from build123d import *

# Parameters (mm, degrees)
SKETCH1_W                = 16.6
SKETCH1_H                = 11.5
BOSS_EXTRUDE1_DEPTH      = 10
SKETCH2_W                = 21
SKETCH2_H                = 14.8
BOSS_EXTRUDE2_DEPTH      = 1.5
SKETCH3_W                = 0.5
SKETCH3_H                = 5
BOSS_EXTRUDE3_DEPTH      = 8
SKETCH4_W                = 0.5
SKETCH4_H                = 0.4
CUT_EXTRUDE1_DEPTH       = 17.75
BOSS_EXTRUDE4_START      = -5.75
SKETCH5_W                = 0.75
SKETCH5_H                = 2.5
BOSS_EXTRUDE4_DEPTH      = 11.5
BOSS_EXTRUDE5_DEPTH      = 2.8
BOSS_EXTRUDE5_DEPTH_BACK = 2.8
CHAMFER1_SIZE            = 1.8
CHAMFER1_SIZE2           = 1.039230485
BOSS_EXTRUDE6_DEPTH      = 4.65
SKETCH9_W                = 1.1
SKETCH9_H                = 0.45
BOSS_EXTRUDE7_DEPTH      = 1.9
CHAMFER2_SIZE            = 0.5
CHAMFER2_SIZE2           = 0.288675135
CHAMFER2_PART_2_SIZE     = 0.5
CHAMFER2_PART_2_SIZE2    = 0.288675135
CHAMFER2_PART_3_SIZE     = 0.5
CHAMFER2_PART_3_SIZE2    = 0.288675135
CHAMFER2_PART_4_SIZE     = 0.5
CHAMFER2_PART_4_SIZE2    = 0.288675135
CHAMFER2_PART_5_SIZE     = 0.5
CHAMFER2_PART_5_SIZE2    = 0.288675135
CHAMFER2_PART_6_SIZE     = 0.5
CHAMFER2_PART_6_SIZE2    = 0.288675135
CHAMFER2_PART_7_SIZE     = 0.5
CHAMFER2_PART_7_SIZE2    = 0.288675135
CHAMFER2_PART_8_SIZE     = 0.5
CHAMFER2_PART_8_SIZE2    = 0.288675135


with BuildPart() as part:
    # Sketch1 → Boss-Extrude1 (new body)
    with BuildSketch(Plane.XY):
        Rectangle(SKETCH1_W, SKETCH1_H)
    extrude(amount=BOSS_EXTRUDE1_DEPTH)

    # Sketch2 → Boss-Extrude2 (add)
    with BuildSketch(Plane.XY.offset(10)):
        Rectangle(SKETCH2_W, SKETCH2_H)
    extrude(amount=BOSS_EXTRUDE2_DEPTH)

    # Sketch3 → Boss-Extrude3 (add)
    with BuildSketch(Plane(origin=(0, 0, 0), x_dir=(-1, 0, 0), z_dir=(0, 0, -1))):
        with Locations((-6, 0)):
            Rectangle(SKETCH3_W, SKETCH3_H)
        Rectangle(SKETCH3_W, SKETCH3_H)
    extrude(amount=BOSS_EXTRUDE3_DEPTH)

    # Sketch4 → Cut-Extrude1 (cut, through all)
    with BuildSketch(Plane(origin=(6.25, 0, 0), x_dir=(0, 0, -1), z_dir=(1, 0, 0))):
        with Locations((2.25, 2.3)):
            Rectangle(SKETCH4_W, SKETCH4_H)
        with BuildLine():
            Line((0, 0.75), (0, -0.75))
            ThreePointArc((0, -0.75), (0.75, 0), (0, 0.75))
        make_face()
        Polygon((6.5, 2.5), (8, 1.449688693), (8, 2.5), align=None)
        with BuildLine():
            Line((5.432692308, 0.612598863), (6.3, 0))
            Line((6.3, 0), (5.432692308, -0.612598863))
            ThreePointArc((5.432692308, -0.612598863), (4.25, 0), (5.432692308, 0.612598863))
        make_face()
        Polygon((8, -2.5), (8, -1.449688693), (6.5, -2.5), align=None)
        with Locations((2.25, -2.3)):
            Rectangle(SKETCH4_W, SKETCH4_H)
    extrude(amount=-CUT_EXTRUDE1_DEPTH, mode=Mode.SUBTRACT)

    # Sketch5 → Boss-Extrude4 (add)
    with BuildSketch(Plane(origin=(0, 0, 0), x_dir=(1, 0, 0), z_dir=(0, 1, 0)).offset(BOSS_EXTRUDE4_START)):
        with Locations((-8.675, -1.25)):
            Rectangle(SKETCH5_W, SKETCH5_H)
    boss_extrude4 = extrude(amount=BOSS_EXTRUDE4_DEPTH)

    # Mirror1: Boss-Extrude4 across plane
    add(boss_extrude4.mirror(Plane(origin=(0, 0, 0), x_dir=(0, 0, 1), z_dir=(1, 0, 0))))

    # Sketch6 → Boss-Extrude5 (add, two sides)
    with BuildSketch(Plane(origin=(0, 0, 0), x_dir=(1, 0, 0), z_dir=(0, 1, 0))) as boss_extrude5_sk:
        with BuildLine():
            Line((-9.05, -2.5), (-10.124907983, -5.653347952))
            ThreePointArc((-10.124907983, -5.653347952), (-10.231819447, -6.312838644), (-10.115557515, -6.970745323))
            Line((-10.115557515, -6.970745323), (-9.056614332, -9.938626949))
            Line((-9.056614332, -9.938626949), (-9.034716365, -10))
            Line((-9.034716365, -10), (-8.3, -10))
            Line((-8.3, -10), (-8.3, -9.827371619))
            Line((-8.3, -9.827371619), (-8.350231447, -9.686588817))
            Line((-8.350231447, -9.686588817), (-9.438479941, -6.636573707))
            ThreePointArc((-9.438479941, -6.636573707), (-9.496610907, -6.307620368), (-9.443155175, -5.977875022))
            Line((-9.443155175, -5.977875022), (-8.34011069, -2.741985882))
            Line((-8.34011069, -2.741985882), (-8.3, -2.624317241))
            Line((-8.3, -2.624317241), (-8.3, -2.5))
            Line((-8.3, -2.5), (-9.05, -2.5))
        make_face()
        with BuildLine():
            Line((8.3, -9.827371619), (8.350231447, -9.686588817))
            Line((8.350231447, -9.686588817), (9.438479941, -6.636573707))
            ThreePointArc((9.438479941, -6.636573707), (9.496610907, -6.307620368), (9.443155175, -5.977875022))
            Line((9.443155175, -5.977875022), (8.34011069, -2.741985882))
            Line((8.34011069, -2.741985882), (8.3, -2.624317241))
            Line((8.3, -2.624317241), (8.3, -2.5))
            Line((8.3, -2.5), (9.05, -2.5))
            Line((9.05, -2.5), (10.124907983, -5.653347952))
            ThreePointArc((10.124907983, -5.653347952), (10.231819447, -6.312838644), (10.115557515, -6.970745323))
            Line((10.115557515, -6.970745323), (9.056614332, -9.938626949))
            Line((9.056614332, -9.938626949), (9.034716365, -10))
            Line((9.034716365, -10), (8.3, -10))
            Line((8.3, -10), (8.3, -9.827371619))
        make_face()
    extrude(amount=BOSS_EXTRUDE5_DEPTH)
    extrude(boss_extrude5_sk.sketch, amount=-BOSS_EXTRUDE5_DEPTH_BACK)

    # Chamfer1
    chamfer1_edges = [part.edges().sort_by_distance(p)[0] for p in [
        (10.5, 0, 11.5),
        (0, 7.4, 11.5),
        (-10.5, 0, 11.5),
        (0, -7.4, 11.5),
    ]]
    chamfer1_side = [part.faces().sort_by_distance(p)[0] for p in [
        (0, 0, 11.5),
    ]]
    chamfer(chamfer1_edges, length=CHAMFER1_SIZE, length2=CHAMFER1_SIZE2, reference=chamfer1_side[0])

    # Sketch7 → Boss-Extrude6 (add, symmetric)
    with BuildSketch(Plane(origin=(0, 0, 0), x_dir=(1, 0, 0), z_dir=(0, 1, 0))):
        with BuildLine():
            Line((-7.2, -11.5), (-3.398718251, -16.8))
            add(Edge.make_bspline(
                [(-3.398718251, -16.8), (0.927387699, -12.334784825), (7.2, -11.5)],
                knots=[0, 0, 0, 1, 1, 1], degree=2))
            Line((7.2, -11.5), (-7.2, -11.5))
        make_face()
    extrude(amount=BOSS_EXTRUDE6_DEPTH, both=True)

    # Sketch9 → Boss-Extrude7 (add)
    with BuildSketch(Plane(origin=(0, 0, 10), x_dir=(-1, 0, 0), z_dir=(0, 0, -1))):
        with Locations((-7.425, 5.975)):
            Rectangle(SKETCH9_W, SKETCH9_H)
        with Locations((-2.475, 5.975)):
            Rectangle(SKETCH9_W, SKETCH9_H)
        with Locations((2.475, 5.975)):
            Rectangle(SKETCH9_W, SKETCH9_H)
        with Locations((7.425, 5.975)):
            Rectangle(SKETCH9_W, SKETCH9_H)
        with Locations((7.425, -5.975)):
            Rectangle(SKETCH9_W, SKETCH9_H)
        with Locations((2.475, -5.975)):
            Rectangle(SKETCH9_W, SKETCH9_H)
        with Locations((-2.475, -5.975)):
            Rectangle(SKETCH9_W, SKETCH9_H)
        with Locations((-7.425, -5.975)):
            Rectangle(SKETCH9_W, SKETCH9_H)
    extrude(amount=BOSS_EXTRUDE7_DEPTH)

    # Chamfer2
    chamfer2_edges = [part.edges().sort_by_distance(p)[0] for p in [
        (7.425, 6.2, 8.1),
    ]]
    chamfer2_side = [part.faces().sort_by_distance(p)[0] for p in [
        (7.425, 6.2, 9.05),
    ]]
    chamfer(chamfer2_edges, length=CHAMFER2_SIZE, length2=CHAMFER2_SIZE2, reference=chamfer2_side[0])

    # Chamfer2 part 2
    chamfer2_part_2_edges = [part.edges().sort_by_distance(p)[0] for p in [
        (2.475, 6.2, 8.1),
    ]]
    chamfer2_part_2_side = [part.faces().sort_by_distance(p)[0] for p in [
        (2.475, 6.2, 9.05),
    ]]
    chamfer(chamfer2_part_2_edges, length=CHAMFER2_PART_2_SIZE, length2=CHAMFER2_PART_2_SIZE2, reference=chamfer2_part_2_side[0])

    # Chamfer2 part 3
    chamfer2_part_3_edges = [part.edges().sort_by_distance(p)[0] for p in [
        (-2.475, 6.2, 8.1),
    ]]
    chamfer2_part_3_side = [part.faces().sort_by_distance(p)[0] for p in [
        (-2.475, 6.2, 9.05),
    ]]
    chamfer(chamfer2_part_3_edges, length=CHAMFER2_PART_3_SIZE, length2=CHAMFER2_PART_3_SIZE2, reference=chamfer2_part_3_side[0])

    # Chamfer2 part 4
    chamfer2_part_4_edges = [part.edges().sort_by_distance(p)[0] for p in [
        (-7.425, 6.2, 8.1),
    ]]
    chamfer2_part_4_side = [part.faces().sort_by_distance(p)[0] for p in [
        (-7.425, 6.2, 9.05),
    ]]
    chamfer(chamfer2_part_4_edges, length=CHAMFER2_PART_4_SIZE, length2=CHAMFER2_PART_4_SIZE2, reference=chamfer2_part_4_side[0])

    # Chamfer2 part 5
    chamfer2_part_5_edges = [part.edges().sort_by_distance(p)[0] for p in [
        (-7.425, -6.2, 8.1),
    ]]
    chamfer2_part_5_side = [part.faces().sort_by_distance(p)[0] for p in [
        (-7.425, -6.2, 9.05),
    ]]
    chamfer(chamfer2_part_5_edges, length=CHAMFER2_PART_5_SIZE, length2=CHAMFER2_PART_5_SIZE2, reference=chamfer2_part_5_side[0])

    # Chamfer2 part 6
    chamfer2_part_6_edges = [part.edges().sort_by_distance(p)[0] for p in [
        (-2.475, -6.2, 8.1),
    ]]
    chamfer2_part_6_side = [part.faces().sort_by_distance(p)[0] for p in [
        (-2.475, -6.2, 9.05),
    ]]
    chamfer(chamfer2_part_6_edges, length=CHAMFER2_PART_6_SIZE, length2=CHAMFER2_PART_6_SIZE2, reference=chamfer2_part_6_side[0])

    # Chamfer2 part 7
    chamfer2_part_7_edges = [part.edges().sort_by_distance(p)[0] for p in [
        (2.475, -6.2, 8.1),
    ]]
    chamfer2_part_7_side = [part.faces().sort_by_distance(p)[0] for p in [
        (2.475, -6.2, 9.05),
    ]]
    chamfer(chamfer2_part_7_edges, length=CHAMFER2_PART_7_SIZE, length2=CHAMFER2_PART_7_SIZE2, reference=chamfer2_part_7_side[0])

    # Chamfer2 part 8
    chamfer2_part_8_edges = [part.edges().sort_by_distance(p)[0] for p in [
        (7.425, -6.2, 8.1),
    ]]
    chamfer2_part_8_side = [part.faces().sort_by_distance(p)[0] for p in [
        (7.425, -6.2, 9.05),
    ]]
    chamfer(chamfer2_part_8_edges, length=CHAMFER2_PART_8_SIZE, length2=CHAMFER2_PART_8_SIZE2, reference=chamfer2_part_8_side[0])


solid = part.part
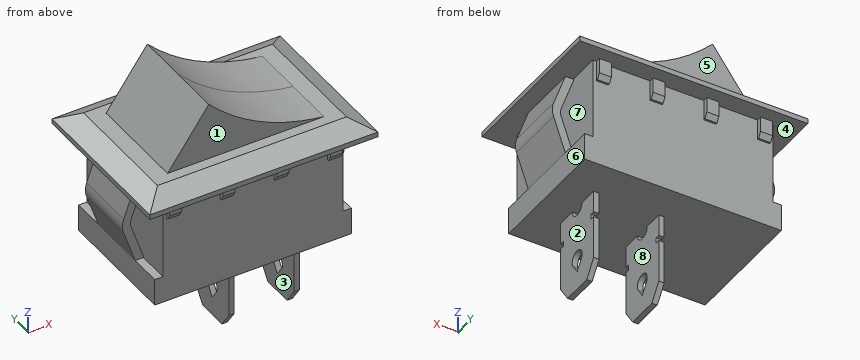
Source: CAD feature listing. Evaluate the final solid. Frame: model axes, mm. Face numbers are marked on the shaded views. A direction names the side the tool comes from. Coordinates: 2 decimals unless noted, no trailing zeros. Loops run counter-clockwise (first coordinate to the right, second up) from the corner with the lowest first, then second, coordinate; pieces in that order, holes last. Notation, with made-up numbers: (76.5, 80.5) -> (102.5, 80.5) arc R9 cw to (102.5, 89.5) -> close; hole circle Ø4 at (85, 59.25). An arc over 180 degrees is marked (long way). Answer in a Markdown table with one row per item. Add a question column.
Q1. Section A-A on z = -5. Return the cut outline in (x, y), and give its area (3 significant figures).
Q2. Pull-direction query (X, two-part tool) for the marked faces 5, 6, 7 and 8; classes: pulls with the +X half, pulls with the -X half, needs draft (parallel to the pull), parting line crosses it, or undercut.
Q3. Section B-B on x = 7.5. Return the cut outline in (y, z), and give its area (3 significant figures).
Q4. Ray query, line 1 along X through (y, z) = (6, 9.75) (3 decimals); line 2 along Y through (x, z) = (0.15, -5); line 3 along Z through (x, y) = (8.5, -4.75). Return the intervals inside material, ascending.
Q5. Contact query for flat-ended pins moving along their axis: pin 1 Ø0.8 at (y, z) = (-1, 0.5) entering from -X; pin 2 Ø8 at (x, z) = (-7, -3) entering from -Y; pin 3 Ø1.5 at (x, z) = (2, 7.5) entering from +Y. Output: stop coordinate, or through.
Q6. Reachability of the marked faces 1, 2, 3 and 4 from +Z, -Z, +X, -X, +Y, -Y: full face, straight path, thin tool, end or side. Return the list, or none.
Computed values:
| question | item | result |
|---|---|---|
| 1 | outline | (-0.25, -2.5) -> (0.25, -2.5) -> (0.25, -0.75) -> (-0.25, -0.75) -> close; (-0.25, 0.75) -> (0.25, 0.75) -> (0.25, 2.5) -> (-0.25, 2.5) -> close; (5.75, -2.5) -> (6.25, -2.5) -> (6.25, -0.75) -> (5.75, -0.75) -> close; (5.75, 0.75) -> (6.25, 0.75) -> (6.25, 2.5) -> (5.75, 2.5) -> close |
| 1 | area | 3.50 mm^2 |
| 2 | face 5 | needs draft |
| 2 | face 6 | pulls with the +X half |
| 2 | face 7 | undercut |
| 2 | face 8 | undercut |
| 3 | outline | (-7.4, 10) -> (-6.2, 10) -> (-6.2, 8.6) -> (-5.91, 8.1) -> (-5.75, 8.1) -> (-5.75, 0) -> (5.75, 0) -> (5.75, 8.1) -> (5.91, 8.1) -> (6.2, 8.6) -> (6.2, 10) -> (7.4, 10) -> (7.4, 10.46) -> (5.6, 11.5) -> (-5.6, 11.5) -> (-7.4, 10.46) -> close |
| 3 | area | 137 mm^2 |
| 4 | line 1 | x = -7.975 to -6.875, -3.025 to -1.925, 1.925 to 3.025, 6.875 to 7.975 |
| 4 | line 2 | y = -2.5 to -0.75, 0.75 to 2.5 |
| 4 | line 3 | z = 0 to 2.5, 10 to 11.5 |
| 5 | pin 1 | stops at x = -9.05 |
| 5 | pin 2 | stops at y = -5.75 |
| 5 | pin 3 | stops at y = 6 |
| 6 | face 1 | +Z, +X, -X, -Y |
| 6 | face 2 | -Z, +X, +Y, -Y |
| 6 | face 3 | -Z, +Y, -Y |
| 6 | face 4 | none |
